```python
from build123d import *

# Parameters (mm, degrees)
SKETCH1_R          = 33.334829616
SKETCH1_R_2        = 12
EXTRUDE1_DEPTH     = 10
SKETCH2_W          = 68.7469374
SKETCH2_H          = 68.7469374
CUT_EXTRUDE1_DEPTH = 10


with BuildPart() as part:
    # Sketch1 → Extrude1 (new body)
    with BuildSketch(Plane(origin=(0, 0, 0), x_dir=(1, 0, 0), z_dir=(0, 1, 0))):
        with Locations(Location((0, 0, 0), (0, 0, 270))):
            Circle(SKETCH1_R)
        with Locations(Location((0, 0, 0), (0, 0, 270))):
            Circle(SKETCH1_R_2, mode=Mode.SUBTRACT)
    extrude(amount=EXTRUDE1_DEPTH)

    # Sketch2 → Cut-Extrude1 (cut)
    with BuildSketch(Plane.XZ):
        Rectangle(SKETCH2_W, SKETCH2_H)
        Polygon((16.16926222, 21.16926222), (21.16926222, 16.16926222), (21.16926222, -16.16926222), (16.16926222, -21.16926222), (-16.16926222, -21.16926222), (-21.16926222, -16.16926222), (-21.16926222, 16.16926222), (-16.16926222, 21.16926222), align=None, mode=Mode.SUBTRACT)
    extrude(amount=-CUT_EXTRUDE1_DEPTH, mode=Mode.SUBTRACT)


solid = part.part
```
Input: part model. Units: mm. Frame: model coordinates. Coordinates: 2 decimals unless noted, no trailing zeros. Write each loop counter-clockwise with the first axis right and the second up, starting at its lowest first coordinate (ties: lowest second). Pieces come first, ordered by that corner, then holes.
1) Material intervals for line 1 along X through (y, z) = (5.25, 0); line 2 along X through (y, z) = (0.5, -1.5); line 3 along Z through (x, y) = (10.5, 2.75), sorted ascending.
2) Section C-C on y = 6.75. Output: boundary loops of the cut face in (x, z).
3) Section B-B on z = 0. Output: boundary loops of the cut face in (x, y), and give its area (3 significant figures).
4) Section A-A on x = 0. Output: boundary loops of the cut face in (y, z).
5) Mould query, pull axis Z, two halves, no side actions, for faces 1 (the flat face through (-21.169, 5, 0)), 2 (the flat face through (0, 5, 21.169)), 3 (the flat face through (0, 5, -21.169)), 4 (the cylindrical face through (3.604, 4.93, 11.446)). Classes: pulls with the +Z half, pulls with the -Z half, needs draft (parallel to the pull), parting line crosses it, or undercut.
6) Section D-D on z = 17.5. Output: boundary loops of the cut face in (x, y).
Check result:
1. line 1: x = -21.17 to -12, 12 to 21.17
1. line 2: x = -21.17 to -11.91, 11.91 to 21.17
1. line 3: z = -21.17 to -5.81, 5.81 to 21.17
2. outline: (-21.17, -16.17) - (-16.17, -21.17) - (16.17, -21.17) - (21.17, -16.17) - (21.17, 16.17) - (16.17, 21.17) - (-16.17, 21.17) - (-21.17, 16.17) - close; hole circle Ø24 at (0, 0)
3. outline: (-21.17, 0) - (-12, 0) - (-12, 10) - (-21.17, 10) - close; (12, 0) - (21.17, 0) - (21.17, 10) - (12, 10) - close
3. area: 183 mm2
4. outline: (0, -21.17) - (10, -21.17) - (10, -12) - (0, -12) - close; (0, 12) - (10, 12) - (10, 21.17) - (0, 21.17) - close
5. face 1: needs draft
5. face 2: pulls with the +Z half
5. face 3: pulls with the -Z half
5. face 4: undercut
6. outline: (-19.84, 0) - (19.84, 0) - (19.84, 10) - (-19.84, 10) - close
